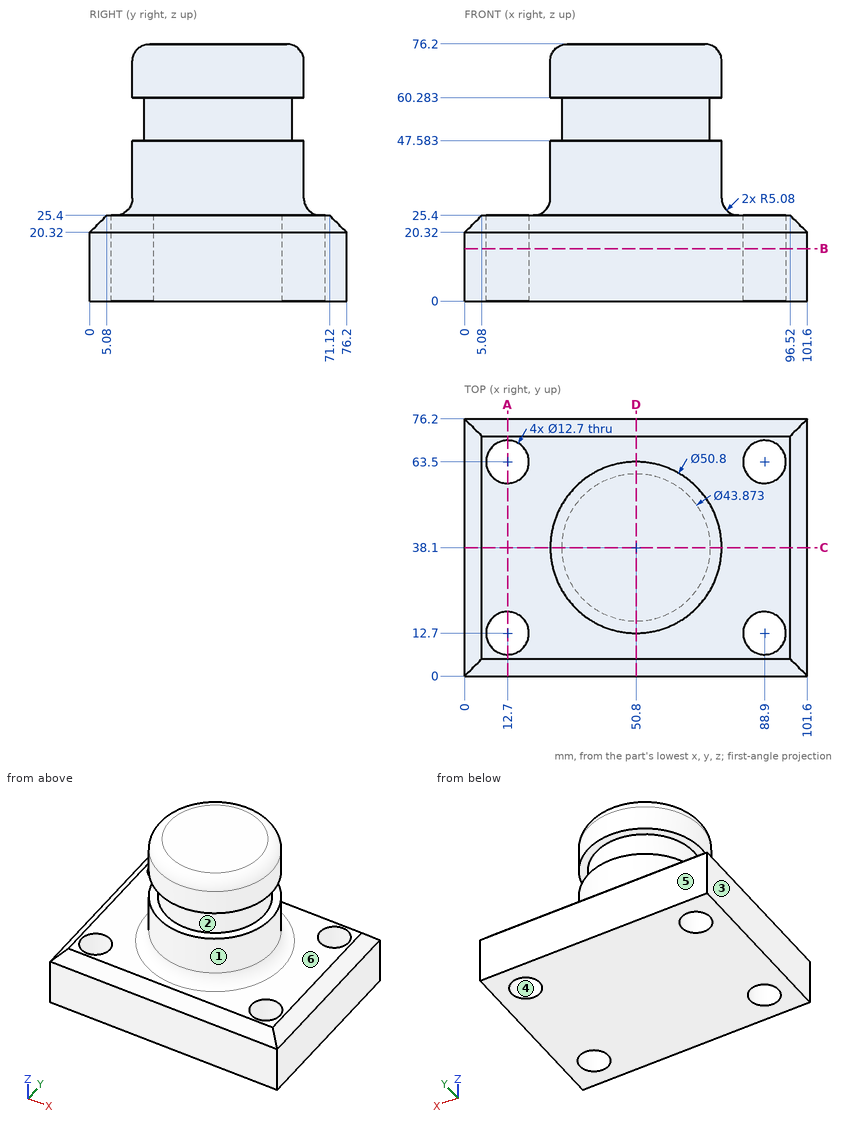
Print and shaded views of the part. All mm, measured from the part's lowest x, y and z. A direction names the side the tool comes from. Coordinates: 2 decimals unless noted, no trailing zeros. Loops run counter-clockwise (first coordinate to the right, second up) from the corner with the lowest first, then second, coordinate; pieces in that order, holes last. Notation, with made-up numbers: (-21, 12.5) - (-7, 12.5) arc R13 ccw to (-7, 27.5) - close; hole circle Ø8 at (-18, 49.5). An arc over 180 degrees is marked (long way). Write item = value, one per line. Start each with the question number.
Item 1: Cut at A-A, the plane x = 12.7. Give the cut face in (y, z).
Item 2: 3-axis set-ups, long thin cutter, end or side, ignore diameter. For the marked faces 1, 2 and 3: which of +Z, -Z, +X, -X, +Y, -Y reach the whole face in a straight line?
Item 3: Mould opens along Y. For the marked faces 4, 5 and 6 say: released by +Y, released by -Y, zero draft, split by the parting line, or undercut.
Item 4: Flat gauge pins, fed straight in: pin 1 Ø16.5 at (x, y) = (88.9, 12.7) entering from -Z; pin 2 Ø10 at (x, y) = (12.7, 63.5) entering from -Z; pin 3 Ø12 at (x, y) = (21, 44.5) entering from +Z (1 decimal); pin 4 Ø6 at (y, z) = (44, 29) entering from -X (1 decimal). Where does each tip first touch, or does it go through?
Item 5: Cut at B-B, the plane z = 15.5. Give the cut face in (x, y).
Item 6: Cut at C-C, the plane y = 38.1. Give the cut face in (x, z).
Item 7: Cut at D-D, the plane x = 50.8. Give the cut face in (y, z), and give its area (3 significant figures).
Item 8: Wall check: L1, parallel to Y at x = 12.7, z = 10; L2, parallel to X at y = 63, z = 11; L3, parallel to Z at x = 62, y = 66.5. Give the ranges that are in metal, low to high. Write a range as from..to.
The answers:
q1.outline = (0, 0) - (6.35, 0) - (6.35, 25.4) - (5.08, 25.4) - (0, 20.32) - close; (19.05, 0) - (57.15, 0) - (57.15, 25.4) - (19.05, 25.4) - close; (69.85, 0) - (76.2, 0) - (76.2, 20.32) - (71.12, 25.4) - (69.85, 25.4) - close
q2.face_1 = +Z
q2.face_2 = none
q2.face_3 = +Z, -Z, -X, +Y, -Y
q3.face_4 = undercut
q3.face_5 = released by +Y
q3.face_6 = zero draft
q4.pin_1 = 0
q4.pin_2 = through
q4.pin_3 = 74
q4.pin_4 = 23.3
q5.outline = (0, 0) - (101.6, 0) - (101.6, 76.2) - (0, 76.2) - close; hole circle Ø12.7 at (12.7, 12.7); hole circle Ø12.7 at (12.7, 63.5); hole circle Ø12.7 at (88.9, 12.7); hole circle Ø12.7 at (88.9, 63.5)
q6.outline = (0, 0) - (101.6, 0) - (101.6, 20.32) - (96.52, 25.4) - (81.28, 25.4) arc R5.08 cw to (76.2, 30.48) - (76.2, 47.58) - (72.74, 47.58) - (72.74, 60.28) - (76.2, 60.28) - (76.2, 71.12) arc R5.08 ccw to (71.12, 76.2) - (30.48, 76.2) arc R5.08 ccw to (25.4, 71.12) - (25.4, 60.28) - (28.86, 60.28) - (28.86, 47.58) - (25.4, 47.58) - (25.4, 30.48) arc R5.08 cw to (20.32, 25.4) - (5.08, 25.4) - (0, 20.32) - close
q7.outline = (0, 0) - (76.2, 0) - (76.2, 20.32) - (71.12, 25.4) - (68.58, 25.4) arc R5.08 cw to (63.5, 30.48) - (63.5, 47.58) - (60.04, 47.58) - (60.04, 60.28) - (63.5, 60.28) - (63.5, 71.12) arc R5.08 ccw to (58.42, 76.2) - (17.78, 76.2) arc R5.08 ccw to (12.7, 71.12) - (12.7, 60.28) - (16.16, 60.28) - (16.16, 47.58) - (12.7, 47.58) - (12.7, 30.48) arc R5.08 cw to (7.62, 25.4) - (5.08, 25.4) - (0, 20.32) - close
q7.area = 4,400 mm2
q8.L1 = 0..6.35, 19.05..57.15, 69.85..76.2
q8.L2 = 0..6.37, 19.03..82.57, 95.23..101.6
q8.L3 = 0..25.4
